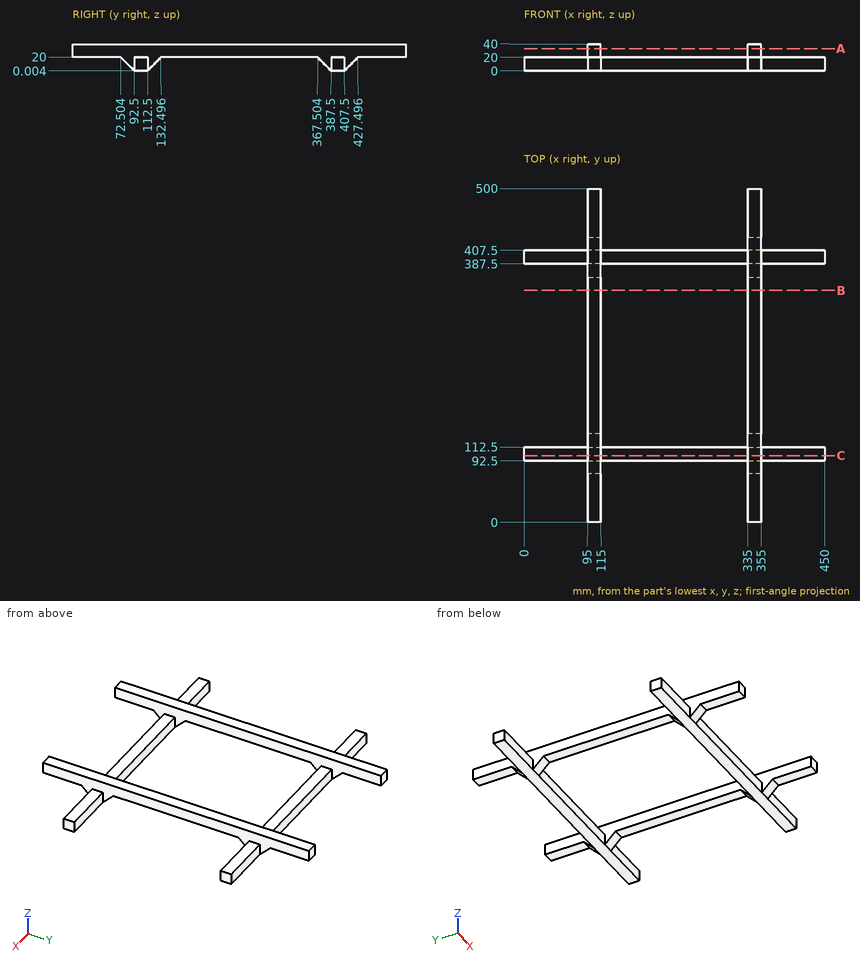
Here's the drawing with two shaded views (mm, measured from the low corner). I have some questions. Round coordinates to 2 decimals unless told otherwise and drop trailing zeros. Loops run counter-clockwise (first coordinate to the right, second up) from the corner with the lowest first, then second, coordinate; pieces in that order, holes last. Notation, with made-up numbers: (67, -18) -> (125, -18) arc R8 ccw to (125, -13) -> close; hole circle Ø5 at (59.25, -40). An arc over 180 degrees is marked (long way). Answer as CSV lines item,"result". Start each with the question number.
1. Imagine slicing it at A-A on z = 33. Write out the boundary of the cut face in (x, y).
2. I'm going to push flat-ended pins straight in: P1, Ø16, axis at x = 271, y = 98, coming from the +Z side; P2, Ø22, axis at x = 348.5, y = 33.5, coming from the -Z side; P3, Ø22, axis at x = 128, z = 10, coming from the +Y side. Where does each tip first touch, or does it pass through?
3. I need wall thicknesses on probe 1 along Y at (x, z) = (377, 11); probe 2 along X at (y, z) = (427, 21); probe 3 along Z at (x, y) = (416, 98.5). Which ranges of each line are inside material? Lowest first, please. Write a range as from..to.
4. Imagine slicing it at B-B on y = 347.5. Write out the boundary of the cut face in (x, z), plus the area to 3 significant figures.
5. Imagine slicing it at C-C on y = 100. Write out the boundary of the cut face in (x, z).
Solution:
1,outline,"(95, 0) -> (115, 0) -> (115, 500) -> (95, 500) -> close; (335, 0) -> (355, 0) -> (355, 500) -> (335, 500) -> close"
2,P1,"z = 20"
2,P2,"z = 20"
2,P3,"y = 407.5"
3,probe 1,"92.5..112.5, 387.5..407.5"
3,probe 2,"95..115, 335..355"
3,probe 3,"0..20"
4,outline,"(95, 20) -> (115, 20) -> (115, 40) -> (95, 40) -> close; (335, 20) -> (355, 20) -> (355, 40) -> (335, 40) -> close"
4,area,"800 mm²"
5,outline,"(0, 0) -> (450, 0) -> (450, 20) -> (355, 20) -> (355, 40) -> (335, 40) -> (335, 20) -> (115, 20) -> (115, 40) -> (95, 40) -> (95, 20) -> (0, 20) -> close"
